from build123d import *

# Parameters (mm, degrees)
SKETCH1_W           = 20
SKETCH1_H           = 40
BOSS_EXTRUDE1_DEPTH = 180
SKETCH2_W           = 20
SKETCH2_H           = 155
CUT_EXTRUDE1_DEPTH  = 29
SKETCH3_W           = 10
SKETCH3_H           = 77.5
CUT_EXTRUDE2_DEPTH  = 29
SKETCH4_W           = 10
SKETCH4_H           = 80
CUT_EXTRUDE3_DEPTH  = 49
SKETCH5_W           = 5
SKETCH5_H           = 77.5
CUT_EXTRUDE4_DEPTH  = 49
SKETCH6_W           = 5
SKETCH6_H           = 77.5
CUT_EXTRUDE5_DEPTH  = 49
SKETCH7_R           = 5
CUT_EXTRUDE6_DEPTH  = 49
SKETCH8_R           = 8
CUT_EXTRUDE7_DEPTH  = 49


with BuildPart() as part:
    # Sketch1 → Boss-Extrude1 (new body)
    with BuildSketch(Plane(origin=(0, 0, 0), x_dir=(1, 0, 0), z_dir=(0, 1, 0))):
        with Locations((10, 20)):
            Rectangle(SKETCH1_W, SKETCH1_H)
    extrude(amount=BOSS_EXTRUDE1_DEPTH)

    # Sketch2 → Cut-Extrude1 (cut)
    with BuildSketch(Plane.ZY):
        with Locations((-10, 102.5)):
            Rectangle(SKETCH2_W, SKETCH2_H)
    extrude(amount=-CUT_EXTRUDE1_DEPTH, mode=Mode.SUBTRACT)

    # Sketch3 → Cut-Extrude2 (cut)
    with BuildSketch(Plane.ZY):
        with Locations((-25, 141.25)):
            Rectangle(SKETCH3_W, SKETCH3_H)
    extrude(amount=-CUT_EXTRUDE2_DEPTH, mode=Mode.SUBTRACT)

    # Sketch4 → Cut-Extrude3 (cut)
    with BuildSketch(Plane(origin=(0, 0, -40), x_dir=(-1, 0, 0), z_dir=(0, 0, -1))):
        with Locations((-10, 40)):
            Rectangle(SKETCH4_W, SKETCH4_H)
    extrude(amount=-CUT_EXTRUDE3_DEPTH, mode=Mode.SUBTRACT)

    # Sketch5 → Cut-Extrude4 (cut)
    with BuildSketch(Plane.XY.offset(-30)):
        with Locations((2.5, 141.25)):
            Rectangle(SKETCH5_W, SKETCH5_H)
    extrude(amount=-CUT_EXTRUDE4_DEPTH, mode=Mode.SUBTRACT)

    # Sketch6 → Cut-Extrude5 (cut)
    with BuildSketch(Plane.XY.offset(-30)):
        with Locations((17.5, 141.25)):
            Rectangle(SKETCH6_W, SKETCH6_H)
    extrude(amount=-CUT_EXTRUDE5_DEPTH, mode=Mode.SUBTRACT)

    # Sketch7 → Cut-Extrude6 (cut)
    with BuildSketch(Plane(origin=(20, 0, 0), x_dir=(0, 0, -1), z_dir=(1, 0, 0))):
        with Locations((10, 10)):
            Circle(SKETCH7_R)
    extrude(amount=-CUT_EXTRUDE6_DEPTH, mode=Mode.SUBTRACT)

    # Sketch8 → Cut-Extrude7 (cut)
    with BuildSketch(Plane(origin=(20, 0, 0), x_dir=(0, 0, -1), z_dir=(1, 0, 0))):
        with Locations((30, 30)):
            Circle(SKETCH8_R)
    extrude(amount=-CUT_EXTRUDE7_DEPTH, mode=Mode.SUBTRACT)


solid = part.part
Source: CAD feature listing. Evaluate the final solid. Frame: model axes, mm. A direction names the side the tool comes from. Coordinates: 2 decimals unless noted, no trailing zeros. Order: outer loops, then holes, each group sorted by start corner. A loop starts at its lowest first (then second) coordinate and runs counter-clockwise, first axis right, second up. Notation, with made-up numbers: M 78.25,88.25 L 92.25,88.25 A16 cw 92.25,116.25 Z; hole C 12.25,87 d1. An arc over 180 degrees is marked long. Write each question's results on one line, items separated by ' | '. Start each with the question number.
Item 1: Cut plane D-D (y = 57.5). Return loops of the section in (x, z).
Item 2: Cut plane C-C (x = 16.75). Return loops of the section in (y, z), and give its area (3 significant figures).
Item 3: First-contact query: pin 1 Ø3 at (x, z) = (9.5, -34) entering from -Y; pin 2 Ø1.5 at (x, z) = (16.5, -28.5) entering from +Y; pin 3 Ø8 at (y, z) = (145.5, -37) entering from -X. Flat tips, straight axial feed; report the tip coordinate or a pass-through.
Item 4: Draft query along X for faces 1 (the face through (2, 12, 0)), 2 (the face through (0, 39, -24)), 3 (the face through (10, 80, -30)), 4 (the face through (5, 39, -25)). Return one class per face: pulls with the +X half, pulls with the -X half, needs draft (parallel to the pull), parting line crosses it, or undercut.
Item 5: Cut plane A-A (y = 30). Return loops of the section in (x, z), and give its area (3 significant figures).
Item 6: Line query: probe 1 along X at (y, z) = (67, -23); probe 2 along Y at (x, z) = (2.2, -10); probe 3 along Y at (x, z) = (5.25, -22.5). Output: solid intervals per line, ascending.
Item 7: Cut plane B-B (z = -10). Return loops of the section in (x, y), and give its area (3 significant figures).
Item 8: Set-up query: faces 5 (the face through (15, 141, -35)), 6 (the face through (15, 39, -25)), 7 (the face through (5, 141, -35)), 8 (the face through (2, 25, -10)). Return all of +Z, -Z, +X, -X, +Y, -Y with unobstructed straight access to the full face (end or side cutting, diameter ignored); none if empty.
Checked values:
1) outline: M 0,-40 L 5,-40 L 5,-20 L 0,-20 Z; M 15,-40 L 20,-40 L 20,-20 L 15,-20 Z
2) outline: M 0,-40 L 102.5,-40 L 102.5,-20 L 25,-20 L 25,0 L 0,0 Z; hole C 10,-10 d10; hole C 30,-30 d16 | area: 2,270 mm2
3) pin 1: stops at y = 80 | pin 2: stops at y = 102.5 | pin 3: stops at x = 5
4) face 1: needs draft | face 2: pulls with the -X half | face 3: undercut | face 4: undercut
5) outline: M 0,-40 L 5,-40 L 5,-38 L 0,-38 Z; M 0,-22 L 5,-22 L 5,-20 L 0,-20 Z; M 15,-40 L 20,-40 L 20,-38 L 15,-38 Z; M 15,-22 L 20,-22 L 20,-20 L 15,-20 Z | area: 40.0 mm2
6) probe 1: x = 0 to 5, 15 to 20 | probe 2: y = 0 to 5, 15 to 25 | probe 3: y = 80 to 102.5
7) outline: M 0,0 L 5,0 L 5,5 L 0,5 Z; M 0,15 L 5,15 L 5,25 L 0,25 Z; M 15,0 L 20,0 L 20,5 L 15,5 Z; M 15,15 L 20,15 L 20,25 L 15,25 Z | area: 150 mm2
8) face 5: +Z, -Z, +X, +Y | face 6: +Z, -Z, -Y | face 7: +Z, -Z, -X, +Y | face 8: +Z, +X, -X, +Y
